Input: part model. Units: mm. Frame: model coordinates. A direction names the side the tool comes from. Give positions to 0.01 mm unless a question says otherwise; leave off trailing zeros. Order: outer loops, then holes, each group sorted by start corner. A loop starts at its lowest first (then second) coordinate and runs counter-clockwise, first axis right, second up. Notation, with made-up numbers: (47.25, 4.25) - (60.25, 4.25) arc R4 cw to (60.25, 11.25) - close; hole circle Ø1 at (37.25, 52). An arc over 180 degrees is marked (long way). Answer in a Markdown table with one row per item. Add a question column.
1. Section query D-D on y = 31.5. Return loops of the section in (x, z).
2. Access query for faces 5 (the face through (35.95, 31.88, 4.68)), 6 (the face through (36, 32, 14.4)). Directions: +Z, -Z, +X, -X, +Y, -Y. A direction counts if a zero-diameter tool reaches every point of the face in a straight line with its end or side. Return the directions, or none.
3. Ray query, line 1 (Y direction, x = 36.5, z = 3); line 2 (Y direction, x = 37, z = 5.5); line 3 (X direction, y = 33.5, z = 7.5). Return the intervals inside material, ascending. Write a range as [from, to].
4. Section query C-C on x = 33.75. Return loops of the section in (y, z).
5. Section query A-A on z = 2. Return loops of the section in (x, y), and give its area (3 significant figures).
6. Mould query, pull axis X, two halves, no side actions, for faces 1 (the face through (31.716, 32, 7)), 2 (the face through (36, 26.6, 7)), 3 (the face through (40.716, 32, 7)), 4 (the face through (36.2, 31.7, 9.5)). Classes: released by +X, released by -X, zero draft, split by the parting line, or undercut.
7. Section query B-B on y = 33.1. Return loops of the section in (x, z), and give its area (3 significant figures).
```python
from build123d import *

# Parameters (mm, degrees)
SKETCH_1_W                               = 9
SKETCH_1_H                               = 11
SKETCH_1_R                               = 3.25
PJ002BH_9X11_FRONT_9P5MM_INSERTION_DEPTH = 9.5
JACK_REAR_BODY_14P4MM_TOTAL_START        = 9.5
SKETCH_2_W                               = 9
SKETCH_2_H                               = 11
JACK_REAR_BODY_14P4MM_TOTAL_DEPTH        = 4.9
SKETCH_3_R                               = 1.25
F_2P5MM_CENTRE_PIN_DEPTH                 = 9.5


with BuildPart() as part:
    # 草图1 → PJ002BH_9x11_front_9p5mm_insertion (new body)
    with BuildSketch(Plane.XY):
        with Locations((36.216, 32.1)):
            Rectangle(SKETCH_1_W, SKETCH_1_H)
        with Locations((36.216, 33.1)):
            Circle(SKETCH_1_R, mode=Mode.SUBTRACT)
    extrude(amount=PJ002BH_9X11_FRONT_9P5MM_INSERTION_DEPTH)

    # 草图2 → Jack_rear_body_14p4mm_total (add)
    with BuildSketch(Plane.XY.offset(JACK_REAR_BODY_14P4MM_TOTAL_START)):
        with Locations((36.216, 32.1)):
            Rectangle(SKETCH_2_W, SKETCH_2_H)
    extrude(amount=JACK_REAR_BODY_14P4MM_TOTAL_DEPTH)

    # 草图3 → 2p5mm_centre_pin (add)
    with BuildSketch(Plane.XY):
        with Locations((36.216, 33.1)):
            Circle(SKETCH_3_R)
    extrude(amount=F_2P5MM_CENTRE_PIN_DEPTH)


solid = part.part
```
Answer:
| question | item | result |
|---|---|---|
| 1 | outline | (31.72, 0) - (33.39, 0) - (33.39, 9.5) - (39.04, 9.5) - (39.04, 0) - (40.72, 0) - (40.72, 14.4) - (31.72, 14.4) - close |
| 2 | face 5 | -Z |
| 2 | face 6 | +Z, +X, -X, +Y, -Y |
| 3 | line 1 | y = [26.6, 29.86], [31.88, 34.32], [36.34, 37.6] |
| 3 | line 2 | y = [26.6, 29.95], [32.13, 34.07], [36.25, 37.6] |
| 3 | line 3 | x = [31.72, 32.99], [35.03, 37.4], [39.44, 40.72] |
| 4 | outline | (26.6, 0) - (30.98, 0) - (30.98, 9.5) - (35.22, 9.5) - (35.22, 0) - (37.6, 0) - (37.6, 14.4) - (26.6, 14.4) - close |
| 5 | outline | (31.72, 26.6) - (40.72, 26.6) - (40.72, 37.6) - (31.72, 37.6) - close; circle Ø2.5 at (36.22, 33.1); hole circle Ø6.5 at (36.22, 33.1) |
| 5 | area | 70.7 mm² |
| 6 | face 1 | released by -X |
| 6 | face 2 | zero draft |
| 6 | face 3 | released by +X |
| 6 | face 4 | undercut |
| 7 | outline | (31.72, 0) - (32.97, 0) - (32.97, 9.5) - (34.97, 9.5) - (34.97, 0) - (37.47, 0) - (37.47, 9.5) - (39.47, 9.5) - (39.47, 0) - (40.72, 0) - (40.72, 14.4) - (31.72, 14.4) - close |
| 7 | area | 91.6 mm² |
